Part model, mm, in its own coordinate system. Face numbers are marked on the shaded views. Give positions to 0.01 mm unless a question says otherwise; leave off trailing zeros. Loops run counter-clockwise (first coordinate to the right, second up) from the corner with the lowest first, then second, coordinate; pieces in that order, holes last. Notation, with made-up numbers: (-11, -8.75) -> (-5, -8.75) arc R19 ccw to (-5, -2.75) -> close; hole circle Ø5 at (89, 47.25). An arc over 180 degrees is marked (long way). Write item = value, one per line.
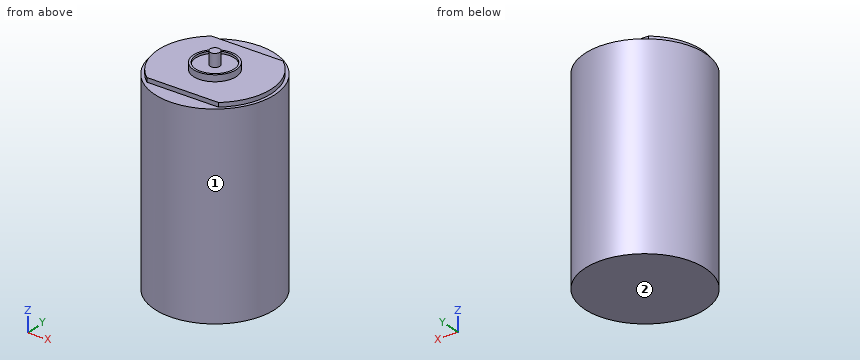
Autodesk Inventor part; units mm, degrees
ref_plane "YZ Plane" through (0, 0, 0) normal (1, 0, 0) x (0, 1, 0)
ref_plane "XZ Plane" through (0, 0, 0) normal (0, 1, 0) x (-1, 0, 0)
ref_plane "XY Plane" through (0, 0, 0) normal (0, 0, 1) x (1, 0, 0)
sketch "Sketch1" plane through (0, 0, 0) normal (0, 0, 1) x (1, 0, 0)
  circle A0 centre (0, 0) radius 14
  dimension "d0" = 28
extrude "Extrusion1" add sketch "Sketch1" along normal blind 46
sketch "Sketch2" plane through (0, 0, 46) normal (0, 0, 1) x (1, 0, 0)
  line L0 (-8.3964, 10.25) -> (8.3964, 10.25)
  line L1 (-8.3964, -10.25) -> (8.3964, -10.25)
  line L2 (-19.6, 0) -> (19.6, 0)
  arc A0 (8.3964, -10.25) -> (8.3964, 10.25) centre (0, 0) ccw
  arc A1 (-8.3964, 10.25) -> (-8.3964, -10.25) centre (0, 0) ccw
  dimension "d4" = 10.25
  dimension "d5" = 10.25
extrude "Extrusion2" add sketch "Sketch2" along normal blind 1
sketch "Sketch3" plane through (0, 0, 47) normal (0, 0, 1) x (1, 0, 0)
  circle A0 centre (0, 0) radius 5
  circle A1 centre (0, 0) radius 4.5
  dimension "d8" = 10
  dimension "d9" = 9
extrude "Extrusion3" add sketch "Sketch3" along normal blind 1.5
sketch "Sketch4" plane through (0, 0, 47) normal (0, 0, 1) x (1, 0, 0)
  circle A0 centre (0, 0) radius 4.5
  dimension "d12" = 9
extrude "Extrusion4" add sketch "Sketch4" along normal blind 1
sketch "Sketch5" plane through (0, 0, 48) normal (0, 0, 1) x (1, 0, 0)
  circle A0 centre (0, 0) radius 1.15
  dimension "d15" = 2.3
extrude "Extrusion5" add sketch "Sketch5" along normal blind 3
properties part number "E600T_RC390_motor_front"
1) Pull direction Y, two halves, no side cores. Call the marked faces 1 and 2: pulls with the +Y half, pulls with the -Y half, needs draft (parallel to the pull), parting line crosses it, or undercut.
Resolved:
face_1 = parting line crosses it
face_2 = needs draft
2) Slice it at C-C, the plane z = 18. List the corners of the cut face in (x, y).
Resolved:
outline = circle Ø28 at (0, 0)
3) Slice it at D-D, the plane y = -6. List the corners of the cut face in (x, z), and give its area (3 significant figures).
Resolved:
outline = (-12.65, 0) -> (12.65, 0) -> (12.65, 46) -> (11.81, 46) -> (11.81, 47) -> (-11.81, 47) -> (-11.81, 46) -> (-12.65, 46) -> close
area = 1,190 mm²
4) Slice it at A-A, the plane y = 0. List the corners of the cut face in (x, z), and give its area (3 significant figures).
Resolved:
outline = (-14, 0) -> (14, 0) -> (14, 46) -> (13.25, 46) -> (13.25, 47) -> (5, 47) -> (5, 48.5) -> (4.5, 48.5) -> (4.5, 48) -> (1.15, 48) -> (1.15, 51) -> (-1.15, 51) -> (-1.15, 48) -> (-4.5, 48) -> (-4.5, 48.5) -> (-5, 48.5) -> (-5, 47) -> (-13.25, 47) -> (-13.25, 46) -> (-14, 46) -> close
area = 1,330 mm²
5) Drop flat-ended pins along their axis: P1, Ø4.5, axis at x = -2, y = 1.5, coming from the +Z side; P2, Ø6, axis at y = -8, z = 34.5, coming from the +X side; P3, Ø5, axis at y = -7, z = 20, coming from the -X side; P4, Ø8, axis at y = -5.5, z = 16.5, coming from the -X side. Give the stop position or say it passes through.
Resolved:
P1 = 51
P2 = 13.08
P3 = -13.26
P4 = -13.92
6) Slice it at B-B, the plane x = 0. List the corners of the cut face in (y, z), and give its area (3 significant figures).
Resolved:
outline = (-14, 0) -> (14, 0) -> (14, 46) -> (10.25, 46) -> (10.25, 47) -> (5, 47) -> (5, 48.5) -> (4.5, 48.5) -> (4.5, 48) -> (1.15, 48) -> (1.15, 51) -> (-1.15, 51) -> (-1.15, 48) -> (-4.5, 48) -> (-4.5, 48.5) -> (-5, 48.5) -> (-5, 47) -> (-10.25, 47) -> (-10.25, 46) -> (-14, 46) -> close
area = 1,330 mm²
7) Drill centre lines: line 1 along Y through (x, z) = (0, 48.35); line 2 along Z through (x, y) = (-1, 2.25); line 3 along Z through (x, y) = (10.5, 6). Where is each one in solid material? Low to high. Write a range as [from, to].
Resolved:
line_1 = [-5, -4.5], [-1.15, 1.15], [4.5, 5]
line_2 = [0, 48]
line_3 = [0, 47]
